Can you work these out from the model? Positions are in its coordinate system, mm. A direction names the side the tool comes from. Round coordinates to 2 decimals unless told otherwise and drop trailing zeros. Order: outer loops, then holes, each group sorted by start corner. A loop starts at its lowest first (then second) coordinate and runs counter-clockwise, first axis right, second up. Notation, with made-up numbers: (72.5, 73.5) -> (99.5, 73.5) arc R22 ccw to (99.5, 82.5) -> close; hole circle Ø9 at (-33, 13). An arc over 180 degrees is marked (long way). Use a Markdown table: item, result. Add a question column.
Q1. We'd pull the mould along X, two halves only. Please class faces 1 (the face through (58.72, -1, -15)), 2 (the face through (44.72, -1, -48)), 3 (the face through (-3, -1, -63.5)): +X half, -X half, draft (parallel to the pull), parting line (faces both ways), or undercut.
Q2. For faces 4 (the face through (12.22, -1, -62)), 5 (the face through (57, -1, -27)), 6 (the face through (-7, 0, -28)), 7 (the face through (-34, -1, -60.5)), which set-ups out of +Z, -Z, +X, -X, +Y, -Y let a thin tool reach every point of the face, with its end or its side?
Q3. If we section it at C-C on y = -1.6: List the corners of the cut face in (x, z) for me, plus the area to 3 significant figures.
Q4. If we section it at B-B on x = 29: List the corners of the cut face in (y, z) for me, plus the area to 3 significant figures.
Q5. I'm going to push flat-ended pins straight in: pin 1 Ø1.5 at (y, z) = (-1, -45.5) entering from +X; pin 2 Ø1.5 at (y, z) = (-1, -62) entering from +X; pin 3 Ø0.9 at (x, y) = (57, -1) entering from -Z. Where does each tip first touch, or does it pass through?
Q6. I need wall thicknesses on line 1 along X through (y, z) = (-1.8, -25); line 2 along Z through (x, y) = (49.5, -1.4); line 3 along Z through (x, y) = (14.5, -2.5). Which ranges of each line are inside material? Lowest first, please. Write a range as [from, to].
Q7. If we section it at D-D on z = -25.5: List the corners of the cut face in (x, y) for me, plus the area to 3 significant figures.
Q8. If we section it at A-A on z = -9: List the corners of the cut face in (x, y) for me.
```python
from build123d import *

# Parameters (mm, degrees)
F0_W     = 30
F0_H     = 3
F1_DEPTH = 3
F2_W     = 3.1
F2_H     = 25
F3_DEPTH = 25
F4_R     = 8
F4_R_2   = 5
F5_DEPTH = 25


with BuildPart() as f1:
    # F0 (on Front) → F1 (new body)
    with BuildSketch(Plane.XZ):
        Polygon((68.720056, 6.5), (44.720056, 6.5), (-50.279944, 6.5), (-53.279944, 6.5), (-53.279944, 0), (-50.279944, -60.5), (-17.779944, -60.5), (12.220056, -60.5), (44.720056, -60.5), (44.720056, -35.5), (68.720056, -35.5), align=None)
        with Locations((-2.779944, -62)):
            Rectangle(F0_W, F0_H)
    extrude(amount=F1_DEPTH)

    # F2 (on face) → F3 (cut)
    with BuildSketch(Plane(origin=(0, 0, 0), x_dir=(-1, 0, 0), z_dir=(0, 1, 0))):
        with Locations((-57.170056, -14.5)):
            Rectangle(F2_W, F2_H)
    extrude(amount=-F3_DEPTH, mode=Mode.SUBTRACT)

    # F4 (on face) → F5 (cut)
    with BuildSketch(Plane.XZ.offset(3)):
        with Locations((-21.452965, -25.5)):
            Circle(F4_R)
        with Locations((4.547035, -25.5)):
            Circle(F4_R)
        with Locations((27.547035, -25.5)):
            Circle(F4_R_2)
    extrude(amount=-F5_DEPTH, mode=Mode.SUBTRACT)


solid = f1.part
```
Answer below:
| question | item | result |
|---|---|---|
| 1 | face 1 | undercut |
| 1 | face 2 | +X half |
| 1 | face 3 | draft |
| 2 | face 4 | -Z, +X, +Y, -Y |
| 2 | face 5 | +Y, -Y |
| 2 | face 6 | +Z, -Z, +X, -X, +Y |
| 2 | face 7 | -Z, -X, +Y, -Y |
| 3 | outline | (-53.28, 0) -> (-50.28, -60.5) -> (-17.78, -60.5) -> (-17.78, -63.5) -> (12.22, -63.5) -> (12.22, -60.5) -> (44.72, -60.5) -> (44.72, -35.5) -> (68.72, -35.5) -> (68.72, 6.5) -> (-53.28, 6.5) -> close; hole circle Ø16 at (-21.45, -25.5); hole circle Ø16 at (4.55, -25.5); hole circle Ø10 at (27.55, -25.5); hole (55.62, -27) -> (58.72, -27) -> (58.72, -2) -> (55.62, -2) -> close |
| 3 | area | 7,020 mm² |
| 4 | outline | (-3, -60.5) -> (0, -60.5) -> (0, -30.28) -> (-3, -30.28) -> close; (-3, -20.72) -> (0, -20.72) -> (0, 6.5) -> (-3, 6.5) -> close |
| 4 | area | 172 mm² |
| 5 | pin 1 | x = 44.72 |
| 5 | pin 2 | x = 12.22 |
| 5 | pin 3 | z = -35.5 |
| 6 | line 1 | [-52.04, -29.44], [-13.47, -3.44], [12.53, 22.57], [32.52, 55.62], [58.72, 68.72] |
| 6 | line 2 | [-35.5, 6.5] |
| 6 | line 3 | [-60.5, 6.5] |
| 7 | outline | (-52.02, -3) -> (-29.45, -3) -> (-29.45, 0) -> (-52.02, 0) -> close; (-13.45, -3) -> (-3.45, -3) -> (-3.45, 0) -> (-13.45, 0) -> close; (12.55, -3) -> (22.55, -3) -> (22.55, 0) -> (12.55, 0) -> close; (32.55, -3) -> (55.62, -3) -> (55.62, 0) -> (32.55, 0) -> close; (58.72, -3) -> (68.72, -3) -> (68.72, 0) -> (58.72, 0) -> close |
| 7 | area | 227 mm² |
| 8 | outline | (-52.83, -3) -> (55.62, -3) -> (55.62, 0) -> (-52.83, 0) -> close; (58.72, -3) -> (68.72, -3) -> (68.72, 0) -> (58.72, 0) -> close |
